```python
from build123d import *

# Parameters (mm, degrees)
HALFBODY_DEPTH                 = 25
CORNERHOLESGUIDE_R             = 12.8
CORNERHOLES_DEPTH              = 12.8
PATTERNCORNERHOLES_COUNT       = 2
PATTERNCORNERHOLES_PITCH       = 130
PATTERNCORNERHOLES_COUNT_DIR2  = 2
PATTERNCORNERHOLES_PITCH_DIR2  = 250
CENTERHOLESGUIDE_R             = 12.8
CENTERHOLES_DEPTH              = 12.8
PATTERNCENTERHOLES_COUNT       = 6
PATTERNCENTERHOLES_PITCH       = 50
CBORE_FOR_M6_SHCS1_D           = 6.6
CBORE_FOR_M6_SHCS1_CBORE_D     = 11.8
CBORE_FOR_M6_SHCS1_CBORE_DEPTH = 6


with BuildPart() as part:
    # Base → HalfBody (new body)
    with BuildSketch(Plane.XY):
        with BuildLine():
            Line((-25, 100), (-25, -100))
            Line((-25, -100), (-100, -100))
            Line((-100, -100), (-100, -150))
            Line((-100, -150), (-7.5, -150))
            ThreePointArc((-7.5, -150), (0, -157.5), (7.5, -150))
            Line((7.5, -150), (100, -150))
            Line((100, -150), (100, -100))
            Line((100, -100), (25, -100))
            Line((25, -100), (25, 100))
            Line((25, 100), (100, 100))
            Line((100, 100), (100, 150))
            Line((100, 150), (7.5, 150))
            ThreePointArc((7.5, 150), (0, 157.5), (-7.5, 150))
            Line((-7.5, 150), (-100, 150))
            Line((-100, 150), (-100, 100))
            Line((-100, 100), (-25, 100))
        make_face()
    extrude(amount=HALFBODY_DEPTH)

    # CornerHolesGuide → CornerHoles (cut)
    with BuildSketch(Plane.XY.offset(25)):
        with Locations((-65, 125)):
            Circle(CORNERHOLESGUIDE_R)
    cornerholes = extrude(amount=-CORNERHOLES_DEPTH, mode=Mode.SUBTRACT)

    # PatternCornerHoles: CornerHoles 2 × 2
    with Locations(*[(i * PATTERNCORNERHOLES_PITCH, -j * PATTERNCORNERHOLES_PITCH_DIR2, 0) for i in range(PATTERNCORNERHOLES_COUNT) for j in range(PATTERNCORNERHOLES_COUNT_DIR2) if (i, j) != (0, 0)]):
        add(cornerholes, mode=Mode.SUBTRACT)

    # CenterHolesGuide → CenterHoles (cut)
    with BuildSketch(Plane.XY.offset(25)):
        with Locations((0, 125)):
            Circle(CENTERHOLESGUIDE_R)
    centerholes = extrude(amount=-CENTERHOLES_DEPTH, mode=Mode.SUBTRACT)

    # PatternCenterHoles: CenterHoles ×6
    with Locations(*[(0, -i * PATTERNCENTERHOLES_PITCH, 0) for i in range(1, PATTERNCENTERHOLES_COUNT)]):
        add(centerholes, mode=Mode.SUBTRACT)

    # CBORE for M6 SHCS1 (through all)
    with Locations(Plane(origin=(0, 0, 0), x_dir=(-1, 0, 0), z_dir=(0, 0, -1))):
        with Locations((-90, 125), (-40, 125), (0, 150), (40, 125), (90, 125), (0, 50), (0, 0), (0, -50), (0, -100), (-90, -125), (-40, -125), (40, -125), (90, -125), (0, -150), (0, 100)):
            CounterBoreHole(CBORE_FOR_M6_SHCS1_D / 2, CBORE_FOR_M6_SHCS1_CBORE_D / 2, CBORE_FOR_M6_SHCS1_CBORE_DEPTH)


solid = part.part
```
The model under review builds one solid part; all positions refer to its coordinate system, in mm. A direction names the side the tool comes from. Round coordinates to 2 decimals unless told otherwise and drop trailing zeros. Loops run counter-clockwise (first coordinate to the right, second up) from the corner with the lowest first, then second, coordinate; pieces in that order, holes last.
Item 1: Take a section at C-C (y = -75). Write out the cut boundary in (x, z), then the cut area to 3 significant figures.
Determined:
outline: (-25, 0) - (25, 0) - (25, 25) - (12.8, 25) - (12.8, 12.2) - (-12.8, 12.2) - (-12.8, 25) - (-25, 25) - close
area: 922 mm2
Item 2: Take a section at B-B (y = 50). Write out the cut boundary in (x, z), then the cut area to 3 significant figures.
Determined:
outline: (-25, 0) - (-5.9, 0) - (-5.9, 6) - (-3.3, 6) - (-3.3, 25) - (-25, 25) - close; (3.3, 6) - (5.9, 6) - (5.9, 0) - (25, 0) - (25, 25) - (3.3, 25) - close
area: 1,050 mm2
Item 3: For line 1 (Y direction, x = 90, z = 18.5); line 2 (Y direction, x = -52, z = 17.5); line 3 (X direction, y = 128, z = 8.25), list the stretches that pass through material, from the lowest coordinate up.
Determined:
line 1: y = -150 to -128.3, -121.7 to -100, 100 to 121.7, 128.3 to 150
line 2: y = -150 to -100, 100 to 150
line 3: x = -100 to -91.37, -88.63 to -41.37, -38.63 to 38.63, 41.37 to 88.63, 91.37 to 100
Item 4: For faces 1 (the face through (-90.72, 121.78, 15.63)), 2 (the face through (-66.67, 137.69, 18.69)), 3 (the face through (-3.172, 154.975, 2.958)), list the 3-axis set-ups (+Z, -Z, +X, -X, +Y, -Y) from which the entire face can be reached by the end or side of a thin tool; tool diameter is ignored.
Determined:
face 1: +Z, -Z
face 2: +Z
face 3: -Z
Item 5: Take a section at A-A (z = 9). Give the number of separate pieces and of enclosed holes in the cut face, then the cut area to 3 significant figures.
Determined:
separate pieces: 1
enclosed holes: 15
area: 29,700 mm2
Item 6: Mouldability with a two-part tool opening along X and no side actions: class faces 4 (the face through (39.28, -128.22, 15.63)), 5 (the face through (-24, 2, 0)), 6 (the face through (25, -1, 12)) as released by +X, released by -X, zero draft, split by the parting line, or undercut.
Determined:
face 4: undercut
face 5: zero draft
face 6: released by +X
Item 7: Take a section at D-D (x = -60). Write out the cut boundary in (y, z), then the cut area to 3 significant figures.
Determined:
outline: (-150, 0) - (-100, 0) - (-100, 25) - (-113.22, 25) - (-113.22, 12.2) - (-136.78, 12.2) - (-136.78, 25) - (-150, 25) - close; (100, 0) - (150, 0) - (150, 25) - (136.78, 25) - (136.78, 12.2) - (113.22, 12.2) - (113.22, 25) - (100, 25) - close
area: 1,900 mm2
Item 8: Clearance check with flat-ended pins moving along their axes: pin 1 Ø13 at (x, y) = (-65, -123) entering from +Z; pin 2 Ø15.5 at (x, y) = (-90, 125) entering from +Z; pin 3 Ø4 at (x, z) = (15, 9) entering from +Y; pin 4 Ø4 at (y, z) = (-14.5, 8) entering from +X. State where each tip first meets the part, or that it passes through.
Determined:
pin 1: stops at z = 12.2
pin 2: stops at z = 25
pin 3: stops at y = 150
pin 4: stops at x = 25
